from build123d import *

# Parameters (mm, degrees)
SKETCH1_R           = 120
SKETCH1_R_2         = 15
BOSS_EXTRUDE3_DEPTH = 16


with BuildPart() as part:
    # Sketch1 → Boss-Extrude3 (new body)
    with BuildSketch(Plane.XY):
        Circle(SKETCH1_R)
        Circle(SKETCH1_R_2, mode=Mode.SUBTRACT)
        with BuildLine():
            Line((10, 87.745437009), (10, 33.268151895))
            ThreePointArc((10, 33.268151895), (24.563895563, 24.563895563), (33.268151895, 10))
            Line((33.268151895, 10), (87.745437009, 10))
            ThreePointArc((87.745437009, 10), (95.562828998, 13.763944958), (97.495374355, 22.222323503))
            ThreePointArc((97.495374355, 22.222323503), (70.707777798, 70.707777798), (22.222323503, 97.495374355))
            ThreePointArc((22.222323503, 97.495374355), (13.763944958, 95.562828998), (10, 87.745437009))
        make_face(mode=Mode.SUBTRACT)
        with BuildLine():
            Line((-10, 87.745437009), (-10, 33.268151895))
            ThreePointArc((-10, 33.268151895), (-24.563895563, 24.563895563), (-33.268151895, 10))
            Line((-33.268151895, 10), (-87.745437009, 10))
            ThreePointArc((-87.745437009, 10), (-95.562828998, 13.763944958), (-97.495374355, 22.222323503))
            ThreePointArc((-97.495374355, 22.222323503), (-70.707777798, 70.707777798), (-22.222323503, 97.495374355))
            ThreePointArc((-22.222323503, 97.495374355), (-13.763944958, 95.562828998), (-10, 87.745437009))
        make_face(mode=Mode.SUBTRACT)
        with BuildLine():
            Line((-10, -33.268151895), (-10, -87.745437009))
            ThreePointArc((-10, -87.745437009), (-13.763944958, -95.562828998), (-22.222323503, -97.495374355))
            ThreePointArc((-22.222323503, -97.495374355), (-70.707777798, -70.707777798), (-97.495374355, -22.222323503))
            ThreePointArc((-97.495374355, -22.222323503), (-95.562828998, -13.763944958), (-87.745437009, -10))
            Line((-87.745437009, -10), (-33.268151895, -10))
            ThreePointArc((-33.268151895, -10), (-24.563895563, -24.563895563), (-10, -33.268151895))
        make_face(mode=Mode.SUBTRACT)
        with BuildLine():
            Line((10, -33.268151895), (10, -87.745437009))
            ThreePointArc((10, -87.745437009), (13.763944958, -95.562828998), (22.222323503, -97.495374355))
            ThreePointArc((22.222323503, -97.495374355), (70.707777798, -70.707777798), (97.495374355, -22.222323503))
            ThreePointArc((97.495374355, -22.222323503), (95.562828998, -13.763944958), (87.745437009, -10))
            Line((87.745437009, -10), (33.268151895, -10))
            ThreePointArc((33.268151895, -10), (24.563895563, -24.563895563), (10, -33.268151895))
        make_face(mode=Mode.SUBTRACT)
    extrude(amount=BOSS_EXTRUDE3_DEPTH)


solid = part.part
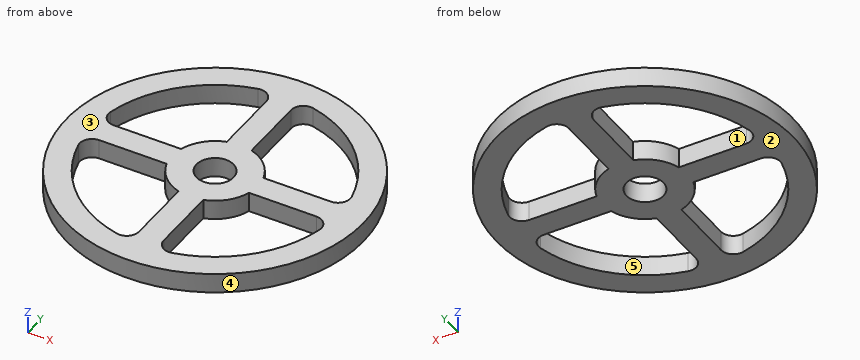
Can you work these out from the model? Positions are in its coordinate system, mm. Face numbers are marked on the shaded views. A direction names the side the tool comes from. Coordinates: 2 decimals unless noted, no trailing zeros. Write each loop counter-clockwise with the first axis right and the second up, starting at its lowest first coordinate (ties: lowest second). Pieces come first, ordered by that corner, then holes. Notation, with made-up numbers: (53.25, 44) -> (76.25, 44) arc R24 ccw to (76.25, 73) -> close; hole circle Ø8 at (-1, 60). An arc over 180 degrees is marked (long way). Write item = value, one per line.
(1) Imagine slicing it at D-D (x = -42.5). Please give me the cut outline in (y, z), and give its area (3 significant figures).
Verdict:
outline = (-112.22, 0) -> (-90.51, 0) -> (-90.51, 16) -> (-112.22, 16) -> close; (-10, 0) -> (10, 0) -> (10, 16) -> (-10, 16) -> close; (90.51, 0) -> (112.22, 0) -> (112.22, 16) -> (90.51, 16) -> close
area = 1,010 mm^2
(2) For pin 1 (18 mm diameter, centred on x = 0, y = 0, fed in from -Z); pin 2 (8 mm diameter, centred on x = -72.5, z = 10, fed in from +Y); pin 3 (5 mm diameter, centred on y = -48.5, z = 11, fed in from -X); pin 4 (1 mm diameter, centred on x = -90, z = 12.5, fed in from -Y), each with a flat end and sliding along its axis, tell me the tip position at first contact or that it passes through.
Verdict:
pin_1 = through
pin_2 = 98.53
pin_3 = -110.83
pin_4 = -79.94
(3) Imagine slicing it at A-A (y = 0). Please give me the cut outline in (x, z), and give its area (3 significant figures).
Verdict:
outline = (-120, 0) -> (-15, 0) -> (-15, 16) -> (-120, 16) -> close; (15, 0) -> (120, 0) -> (120, 16) -> (15, 16) -> close
area = 3,360 mm^2
(4) On a 3-axis mill with a long thin cutter (end or side, diameter ignored), from which of +Z, -Z, +X, -X, +Y, -Y can I reach the whole of each face in a straight line? I mean the marked faces 1 and 2. Say none if no direction works.
Verdict:
face_1 = +Z, -Z
face_2 = -Z, +X, -X, +Y, -Y
(5) Imagine slicing it at C-C (z = 2.5). Please give me the cut outline in (x, y), and give its area (3 significant figures).
Verdict:
outline = circle Ø240 at (0, 0); hole (-97.5, -22.22) arc R100 ccw to (-22.22, -97.5) arc R10 ccw to (-10, -87.75) -> (-10, -33.27) arc R34.74 cw to (-33.27, -10) -> (-87.75, -10) arc R10 ccw to start; hole (-97.5, 22.22) arc R10 ccw to (-87.75, 10) -> (-33.27, 10) arc R34.74 cw to (-10, 33.27) -> (-10, 87.75) arc R10 ccw to (-22.22, 97.5) arc R100 ccw to start; hole circle Ø30 at (0, 0); hole (10, -87.75) arc R10 ccw to (22.22, -97.5) arc R100 ccw to (97.5, -22.22) arc R10 ccw to (87.75, -10) -> (33.27, -10) arc R34.74 cw to (10, -33.27) -> close; hole (10, 33.27) arc R34.74 cw to (33.27, 10) -> (87.75, 10) arc R10 ccw to (97.5, 22.22) arc R100 ccw to (22.22, 97.5) arc R10 ccw to (10, 87.75) -> close
area = 22,400 mm^2
(6) If I drill on probe 1 along Y at (x, z) = (-80.5, 7); probe 2 along X at (y, z) = (36, 2.5); probe 3 along X at (y, z) = (54, 12), over which ranges is the centre line in solid material (lowest first)?
Verdict:
probe_1 = -88.99 to -59.32, -10 to 10, 59.32 to 88.99
probe_2 = -114.47 to -93.29, -10 to 10, 93.29 to 114.47
probe_3 = -107.16 to -84.16, -10 to 10, 84.16 to 107.16
(7) Thinking about a two-plate mould opening in X: for the marked faces 3, 4 and 5, which applies, +X half, -X half, draft (parallel to the pull), parting line (faces both ways), or undercut?
Verdict:
face_3 = draft
face_4 = parting line
face_5 = undercut
